The listing builds one solid part. Answer for the finished solid, in the listing's coordinates (mm). Coordinates: 2 decimals unless noted, no trailing zeros. Order: outer loops, then holes, each group sorted by start corner. A loop starts at its lowest first (then second) coordinate and runs counter-clockwise, first axis right, second up. Notation, with made-up numbers: (84, 71.25) -> (131, 71.25) arc R37 ccw to (131, 109.25) -> close; hole circle Ø3 at (76, 20.25). An arc over 180 degrees is marked (long way). Write item = value, one per line.
from build123d import *

# Parameters (mm, degrees)
F0_R     = 12.5
F2_DEPTH = 100
F1_R     = 3.15
F3_DEPTH = 200
F4_R     = 5


with BuildPart() as f2:
    # F0 (on Front) → F2 (new body, symmetric)
    with BuildSketch(Plane.XZ):
        Circle(F0_R)
    extrude(amount=F2_DEPTH, both=True)

    # F1 (on Right) → F3 (cut, symmetric)
    with BuildSketch(Plane.YZ):
        with Locations((-88, 0)):
            Circle(F1_R)
        with Locations((88, 0)):
            Circle(F1_R)
    extrude(amount=F3_DEPTH, both=True, mode=Mode.SUBTRACT)

    # F4
    f4_edges = [f2.edges().sort_by_distance(p)[0] for p in [
        (-12.5, -100, 0),
        (-12.5, 100, 0),
    ]]
    fillet(f4_edges, radius=F4_R)


solid = f2.part
Q1. The mould has two halves that part along Z. Classify faces 1 (the face through (0, 100, 0)), 2 (the face through (0.171, 84.853, 0.138)), 3 (the face through (11.923, -1.33, 3.755)): released by +Z, released by -Z, zero draft, split by the parting line, or undercut.
The answers:
face_1 = zero draft
face_2 = undercut
face_3 = split by the parting line
Q2. Section A-A, the plane z = 0 is taken. Give the vertices of the cut face in (x, y).
The answers:
outline = (-12.5, -95) arc R5 ccw to (-7.5, -100) -> (7.5, -100) arc R5 ccw to (12.5, -95) -> (12.5, -91.15) -> (-12.5, -91.15) -> close; (-12.5, -84.85) -> (12.5, -84.85) -> (12.5, 84.85) -> (-12.5, 84.85) -> close; (-12.5, 91.15) -> (12.5, 91.15) -> (12.5, 95) arc R5 ccw to (7.5, 100) -> (-7.5, 100) arc R5 ccw to (-12.5, 95) -> close
Q3. Section B-B, the plane y = -42.5 is taken. Give the vertices of the cut face in (x, z), plus the area to 3 significant figures.
The answers:
outline = circle Ø25 at (0, 0)
area = 491 mm2
Q4. Section D-D, the plane y = -88 is taken. Give the vertices of the cut face in (x, z).
The answers:
outline = (-12.1, -3.15) arc R12.5 ccw to (12.1, -3.15) -> close; (-12.1, 3.15) -> (12.1, 3.15) arc R12.5 ccw to start
Q5. Find the intervals of material crossed by line 1 along Y through (x, z) = (-3.5, 0); line 2 along Y through (x, z) = (10, 0); line 3 along Z through (x, y) = (8, -88), in increasing order.
The answers:
line_1 = -100 to -91.15, -84.85 to 84.85, 91.15 to 100
line_2 = -99.33 to -91.15, -84.85 to 84.85, 91.15 to 99.33
line_3 = -9.6 to -3.15, 3.15 to 9.6
Q6. Each of these flat-tipped pins is pushed along its axis until it touches: pin 1 Ø10 at (y, z) = (64, 5.5) entering from -X; pin 2 Ø3 at (x, y) = (5.5, -9.5) entering from +Z; pin 3 Ø6 at (x, z) = (-9, -7.5) entering from -Y. Where does it stop, or does it pass through?
The answers:
pin_1 = -12.49
pin_2 = 11.84
pin_3 = -99.85
Q7. Section C-C, the plane x = 4.5 is taken. Give the number of separate pieces and of enclosed holes in the cut face, plus the area to 3 significant figures.
The answers:
separate_pieces = 1
enclosed_holes = 2
area = 4,580 mm2
